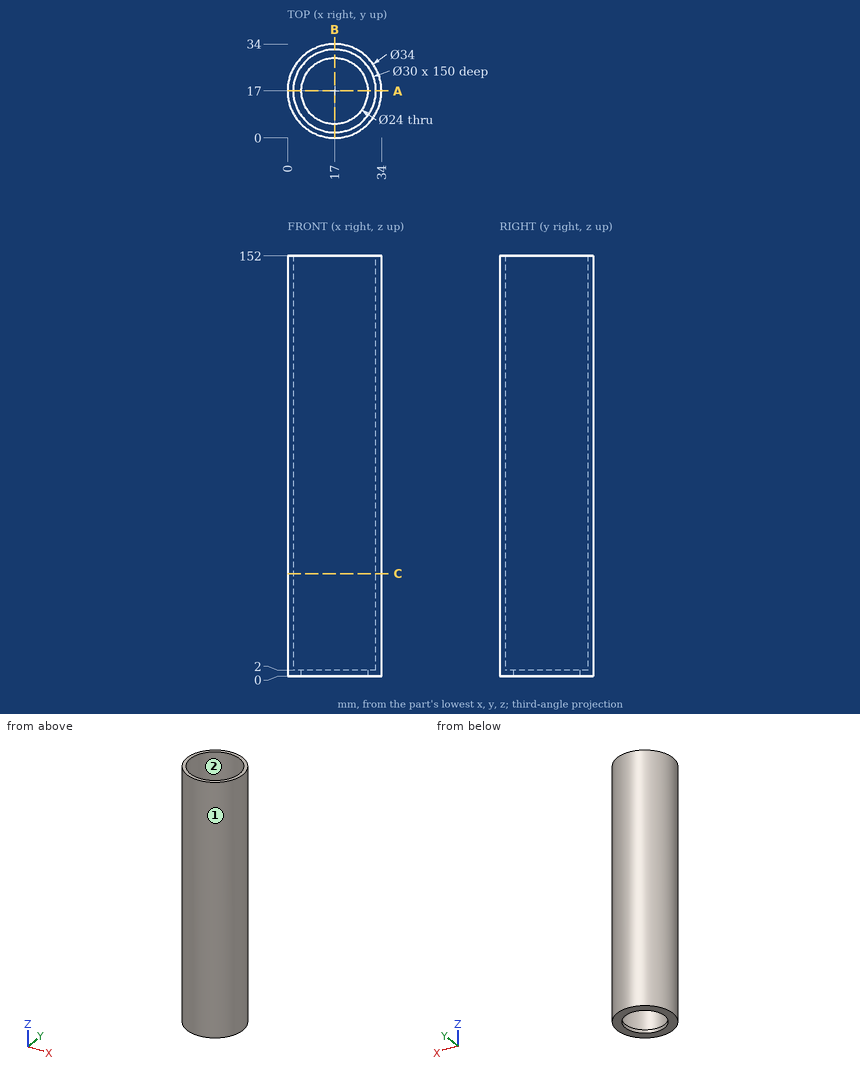
For this review, use the dimensioned drawing (mm, ordinates from the lowest corner) and the shaded views. Coordinates: 2 decimals unless noted, no trailing zeros. Order: outer loops, then holes, each group sorted by start corner. A loop starts at its lowest first (then second) coordinate and runs counter-clockwise, first axis right, second up. Notation, with made-up numbers: (-29.5, 57) - (-11.5, 57) arc R7 ccw to (-11.5, 70) - close; hole circle Ø8 at (56, 6). An arc over 180 degrees is marked (long way). Answer as a JSON object with one key per item and string values. Group by question number.
1. We need section C-C on z = 37. State the section outline as (x, y) points.
2. We need section A-A on y = 17. State the section outline as (x, z) points, then the cut area to 3 significant figures.
3. For probe 1 along Y at (x, z) = (17, 112.5); probe 2 along Y at (x, z) = (17, 0.5); probe 3 along Z at (x, y) = (4, 16.5), list the stretches that pass through material, from the lowest coordinate up.
4. Clearance check with flat-ended pins moving along their axes: P1, Ø3, axis at x = 10.5, z = 35.5, coming from the -Y side; P2, Ø3, axis at y = 23, z = 58, coming from the -X side; P3, Ø2, axis at y = 14, z = 110.5, coming from the -X side. State where each tip first meets the part, or that it passes through.
5. The part is to be moulded in two halves that separate along Y. For the marked faces 1 and 2, say which applies: pulls with the +Y half, pulls with the -Y half, needs draft (parallel to the pull), parting line crosses it, or undercut.
Final values:
{
 "1": {"outline": "circle Ø34 at (17, 17); hole circle Ø30 at (17, 17)"},
 "2": {"outline": "(0, 0) - (5, 0) - (5, 2) - (2, 2) - (2, 152) - (0, 152) - close; (29, 0) - (34, 0) - (34, 152) - (32, 152) - (32, 2) - (29, 2) - close", "area": "620 mm²"},
 "3": {"probe 1": "0 to 2, 32 to 34", "probe 2": "0 to 5, 29 to 34", "probe 3": "0 to 2"},
 "4": {"P1": "y = 0.75", "P2": "x = 0.61", "P3": "x = 0.12"},
 "5": {"face 1": "parting line crosses it", "face 2": "undercut"}
}
